Part model, mm, in its own coordinate system. A direction names the side the tool comes from. Give positions to 0.01 mm unless a question says otherwise; leave off trailing zeros. Order: outer loops, then holes, each group sorted by start corner. A loop starts at its lowest first (then second) coordinate and runs counter-clockwise, first axis right, second up. Notation, with made-up numbers: (37, -4.5) - (79, -4.5) arc R8 cw to (79, 3.5) - close; hole circle Ø3 at (-29, 73.25). An arc over 180 degrees is marked (long way). One line per item, written item: value.
Autodesk Inventor part; units mm, degrees
ref_plane "YZ Plane" through (0, 0, 0) normal (1, 0, 0) x (0, 1, 0)
ref_plane "XZ Plane" through (0, 0, 0) normal (0, 1, 0) x (-1, 0, 0)
ref_plane "XY Plane" through (0, 0, 0) normal (0, 0, 1) x (1, 0, 0)
sketch "Sketch1" plane through (0, 0, 0) normal (1, 0, 0) x (0, 1, 0)
  line L0 (-18.7654, 35.1522) -> (-8.7039, 30.9846)
  line L1 (8.7039, 30.9846) -> (18.7654, 35.1522)
  line L2 (-21, 41) -> (21, 41) construction
  line L3 (-5, 25.4414) -> (-5, 10.198)
  line L4 (5, 25.4414) -> (5, 10.198)
  arc A0 (-5, 25.4414) -> (-8.7039, 30.9846) centre (-11, 25.4414) ccw
  arc A1 (8.7039, 30.9846) -> (5, 25.4414) centre (11, 25.4414) ccw
  arc A2 (-6.6, 6.1188) -> (6.6, 6.1188) centre (0, 0) ccw
  arc A3 (-6.6, 6.1188) -> (-5, 10.198) centre (-11, 10.198) ccw
  arc A4 (5, 10.198) -> (6.6, 6.1188) centre (11, 10.198) ccw
  line L5 (4, 3.3563) -> (4, -3)
  line L6 (3, -4) -> (-3, -4)
  line L7 (-4, -3) -> (-4, 3.3563)
  line L8 (-4, 4) -> (4, -4) construction
  line L9 (4, 4) -> (-4, -4) construction
  arc A5 (1.9545, 13.4242) -> (-1.9545, 13.4242) centre (0, 13) ccw
  line L10 (0, 13) -> (0, 0) construction
  line L11 (-3.8635, 4.629) -> (-1.9545, 13.4242)
  line L12 (3.8635, 4.629) -> (1.9545, 13.4242)
  arc A6 (-3.8635, 4.629) -> (-4, 3.3563) centre (2, 3.3563) ccw
  arc A7 (4, 3.3563) -> (3.8635, 4.629) centre (-2, 3.3563) ccw
  arc A8 (-4, -3) -> (-3, -4) centre (-3, -3) ccw
  arc A9 (3, -4) -> (4, -3) centre (3, -3) ccw
  line L13 (-5, 38) -> (-5, 41)
  line L14 (5.2222, 41) -> (5.2222, 38)
  line L15 (-20, 38) -> (-5, 38)
  line L16 (5.2222, 38) -> (20, 38)
  line L17 (-20, 38) -> (-20, 37)
  line L18 (20, 38) -> (20, 37)
  circle A10 centre (0, 0) radius 46 construction
  arc A11 (-20, 37) -> (-18.7654, 35.1522) centre (-18, 37) ccw
  arc A12 (18.7654, 35.1522) -> (20, 37) centre (18, 37) ccw
  line L19 (-5, 40.9488) -> (5.2222, 40.9409)
  point P0 (-5, 29.4504)
  point P1 (5, 29.4504)
  point P2 (-5, 7.4833)
  point P3 (5, 7.4833)
  point P4 (0, 0)
  dimension "d25" = 10
  dimension "d32" = 6
  dimension "d33" = 6
  dimension "d68" = 18
  dimension "d69" = 6
  dimension "d75" = 8
  dimension "d76" = 8
  dimension "d77" = 4
  dimension "d78" = 13
  dimension "d79" = 6
  dimension "d80" = 1
  dimension "d82" = 46
  dimension "d84" = 38
  dimension "d85" = 3
  dimension "d86" = 5
  dimension "d87" = 20
  dimension "d88" = 40
  dimension "d90" = 2
  dimension "d93" = 1
  dimension "d94" = 1
  dimension "d95" = 22.5
  dimension "d96" = 22.5
  dimension "d97" = 4
  dimension "d98" = 4
extrude "Extrusion6" add sketch "Sketch1" along normal blind 3
properties part number "Camera Mount_B073113"
1) Drop flat-ended pins along their axis: P1, Ø1.5, axis at x = 2, y = -9.5, coming from the +Z side; P2, Ø0.9, axis at x = 1, y = 0.5, coming from the +Z side; P3, Ø1, axis at x = 0.5, z = 3, coming from the +Y side. Give the stop position or say it passes through.
Answer:
P1: stops at z = 38
P2: stops at z = 40.94
P3: stops at y = 8.65
2) Wall check: line 1 along Z through (x, y) = (0.9, -6); line 2 along Z through (x, y) = (1.1, 6.5); line 3 along Y through (x, z) = (2.4, 23.5). Give the ranges that are in metal, low to high. Write a range as [from, to].
Answer:
line 1: z = [-6.71, 6.88], [28.76, 38]
line 2: z = [-6.22, 6.23], [29.41, 38]
line 3: y = [-5, 5]
3) Two-plate mould, pull along Z, no slides. Class faces 1 (the face through (1, 13, 38)), 2 (the face through (0, -2, 20)), 3 (the face through (1.48, -6.04, 28.82)), 4 (the face through (1, 0, -9)): pulls with the +Z half, pulls with the -Z half, needs draft (parallel to the pull), parting line crosses it, or undercut.
Answer:
face 1: pulls with the +Z half
face 2: needs draft
face 3: undercut
face 4: undercut
4) Slice it at C-C on y = 0. Write the cut outline in (x, z), then the cut area to 3 significant figures.
Answer:
outline: (0, -9) - (3, -9) - (3, -4) - (0, -4) - close; (0, 15) - (3, 15) - (3, 40.94) - (0, 40.94) - close
area: 92.8 mm2
5) Slice it at B-B on x = 2. Write the cut outline in (y, z).
Answer:
outline: (-20, 37) arc R2 ccw to (-18.77, 35.15) - (-8.7, 30.98) arc R6 cw to (-5, 25.44) - (-5, 10.2) arc R6 cw to (-6.6, 6.12) arc R9 ccw (long way) to (6.6, 6.12) arc R6 cw to (5, 10.2) - (5, 25.44) arc R6 cw to (8.7, 30.98) - (18.77, 35.15) arc R2 ccw to (20, 37) - (20, 38) - (5.22, 38) - (5.22, 40.94) - (-5, 40.95) - (-5, 38) - (-20, 38) - close; hole (-4, -3) arc R1 ccw to (-3, -4) - (3, -4) arc R1 ccw to (4, -3) - (4, 3.36) arc R6 ccw to (3.86, 4.63) - (1.95, 13.42) arc R2 ccw to (-1.95, 13.42) - (-3.86, 4.63) arc R6 ccw to (-4, 3.36) - close
6) Slice it at D-D on y = -14. Write the cut outline in (x, z), then the cut area to 3 significant figures.
Answer:
outline: (0, 33.18) - (3, 33.18) - (3, 38) - (0, 38) - close
area: 14.5 mm2
7) Which spindle directions (+Z, -Z, +X, -X, +Y, -Y) get a long thin tool onto all of the face, cutting with end or side? Do faces 5 (the face through (1.48, -5.4, 8.04)), 6 (the face through (1, 5.222, 39)), 7 (the face through (1.48, 5.98, 28.73)), 8 (the face through (1.479, 3.965, 4.005)). Say none if no direction does.
Answer:
face 5: +X, -X, -Y
face 6: +Z, +X, -X, +Y
face 7: +X, -X, +Y
face 8: +X, -X
8) Slice it at A-A on z = 0. Write the cut outline in (x, y).
Answer:
outline: (0, -9) - (3, -9) - (3, -4) - (0, -4) - close; (0, 4) - (3, 4) - (3, 9) - (0, 9) - close
